Can you work these out from the model? Positions are in its coordinate system, mm. Face numbers are marked on the shaded views. A direction names the side the tool comes from. Round coordinates to 2 decimals unless told otherwise and drop trailing zeros. Loops run counter-clockwise (first coordinate to the right, second up) from the corner with the lowest first, then second, coordinate; pieces in that order, holes last. Notation, with made-up numbers: (-28.5, -22.75) -> (-23.5, -22.75) arc R9 cw to (-23.5, -5.75) -> close; hole circle Ø3 at (-34.75, 26.5). An arc over 180 degrees is marked (long way). Answer as a JSON object with one key per item and string values.
```python
from build123d import *

# Parameters (mm, degrees)
SKETCH2_W                = 12.7
SKETCH2_H                = 14.91
SKETCH2_R                = 5.08
BOSS_EXTRUDE1_DEPTH      = 9.525
BOSS_EXTRUDE2_START      = 9.525
BOSS_EXTRUDE2_DEPTH      = 6.35
BOSS_EXTRUDE3_DEPTH      = 2
BOSS_EXTRUDE7_START      = -25.4
BOSS_EXTRUDE7_DEPTH      = 50.8
SKETCH5_W                = 9.77111141
SKETCH5_H                = 3
CUT_EXTRUDE1_DEPTH       = 68.279429146
CUT_EXTRUDE2_START       = -12.902497
SKETCH6_W                = 30.31497918
SKETCH6_H                = 2.000002
SKETCH6_W_2              = 22.73097918
SKETCH6_H_2              = 6.646875
CUT_EXTRUDE2_DEPTH       = 12.902497
CUT_EXTRUDE3_START       = 0.499999
SKETCH6_3_W              = 22.73097918
SKETCH6_3_H              = 2.000002
SKETCH6_3_H_2            = 4.646873
SKETCH6_3_W_2            = 0.271399
SKETCH6_3_H_3            = 3
CUT_EXTRUDE3_DEPTH       = 7.0000114
FILLET2_R                = 17.78
CUT_EXTRUDE4_DEPTH       = 33.871006443
CUT_EXTRUDE4_DEPTH_BACK  = 33.871006443
SKETCH7_W                = 10.16
SKETCH7_H                = 10.092503778
FILLET3_R                = 2.54
SKETCH8_W                = 1.515
SKETCH8_H                = 2.54
BOSS_EXTRUDE8_DEPTH      = 2
FILLET4_R                = 5.08
CUT_EXTRUDE5_DEPTH       = 35.535859512
BOSS_EXTRUDE9_DEPTH      = 3.646875
SET_SCREW_CUT_REACH      = 43.018
SET_SCREW_CUT_END_RADIUS = 5.08
SKETCH12_R               = 1.4


# Read off the part's stored shape, not the designer's step: Boss-Extrude7
with BuildPart() as part:
    # Sketch2 → Boss-Extrude1 (new body)
    with BuildSketch(Plane.XY):
        with Locations((0, 7.455)):
            Rectangle(SKETCH2_W, SKETCH2_H)
        with Locations(Location((0, 7.83, 0), (0, 0, 180))):
            Circle(SKETCH2_R, mode=Mode.SUBTRACT)
    extrude(amount=BOSS_EXTRUDE1_DEPTH)

    # Sketch2<3> → Boss-Extrude2 (add)
    with BuildSketch(Plane.XY.offset(BOSS_EXTRUDE2_START)):
        Polygon((2.286, 0), (-2.286, 0), (-2.286, -5.334), (-4.826, -5.334), (-4.826, -14.859), (4.826, -14.859), (4.826, -5.334), (2.286, -5.334), align=None)
    extrude(amount=-BOSS_EXTRUDE2_DEPTH)

    # Sketch3 → Boss-Extrude3 (add)
    with BuildSketch(Plane.XZ):
        Polygon((14.9225, 9.525), (-14.9225, 9.525), (-14.9225, -11.557), (-10.85748959, -11.557), (10.85748959, -11.557), (14.9225, -11.557), align=None)
    extrude(amount=-BOSS_EXTRUDE3_DEPTH)

    # Boss-Extrude7 outline → Boss-Extrude7 (add)
    with BuildSketch(Plane(origin=(0, 0, 0), x_dir=(0, 0, -1), z_dir=(1, 0, 0)).offset(BOSS_EXTRUDE7_START)):
        with BuildLine():
            Line((5.848505491, 2), (11.557, 0))
            Line((11.557, 0), (12.724273166, 0.598024588))
            ThreePointArc((12.724273166, 0.598024588), (12.796184179, 0.55223881), (12.869936616, 0.509482413))
            Line((12.869936616, 0.509482413), (20.955, 3.646875))
            Line((20.955, 3.646875), (23.495, 3.646875))
            Line((23.495, 3.646875), (23.495, 6.646875))
            Line((23.495, 6.646875), (17.823506348, 6.646875))
            Line((17.823506348, 6.646875), (5.848505491, 2))
        make_face()
    extrude(amount=BOSS_EXTRUDE7_DEPTH)

    # Sketch5 → Cut-Extrude1 (cut, through all)
    with BuildSketch(Plane(origin=(0, 37.971305566, -23.495), x_dir=(1, 0, 0), z_dir=(0, 0, 1))):
        Polygon((25.4, -37.971305566), (25.4, -34.324430566), (15.62888859, -34.324430566), (14.9225, -34.324430566), (14.9225, -37.971305566), align=None)
        with Locations((20.514444295, -32.824430566)):
            Rectangle(SKETCH5_W, SKETCH5_H)
        Polygon((-25.4, -34.324430566), (-25.4, -37.971305566), (-14.9225, -37.971305566), (-14.9225, -34.324430566), (-15.62888859, -34.324430566), align=None)
        with Locations((-20.514444295, -32.824430566)):
            Rectangle(SKETCH5_W, SKETCH5_H)
    extrude(amount=CUT_EXTRUDE1_DEPTH, mode=Mode.SUBTRACT)

    # Sketch6 → Cut-Extrude2 (cut)
    with BuildSketch(Plane(origin=(0, 0, -22.995001), x_dir=(-1, 0, 0), z_dir=(0, 0, -1)).offset(CUT_EXTRUDE2_START)):
        with Locations((0, 5.646874)):
            Rectangle(SKETCH6_W, SKETCH6_H)
        with Locations((0, 3.3234375)):
            Rectangle(SKETCH6_W_2, SKETCH6_H_2)
    extrude(amount=CUT_EXTRUDE2_DEPTH, mode=Mode.SUBTRACT)

    # Sketch6<3> → Cut-Extrude3 (cut)
    with BuildSketch(Plane(origin=(0, 0, -22.995001), x_dir=(-1, 0, 0), z_dir=(0, 0, -1)).offset(CUT_EXTRUDE3_START)):
        with Locations((0, 5.646874)):
            Rectangle(SKETCH6_3_W, SKETCH6_3_H)
        with Locations((0, 2.3234365)):
            Rectangle(SKETCH6_3_W, SKETCH6_3_H_2)
        with Locations((-15.49318909, 5.146875)):
            Rectangle(SKETCH6_3_W_2, SKETCH6_3_H_3)
        with Locations((15.49318909, 5.146875)):
            Rectangle(SKETCH6_3_W_2, SKETCH6_3_H_3)
    extrude(amount=-CUT_EXTRUDE3_DEPTH, mode=Mode.SUBTRACT)

    # Fillet2
    fillet2_edges = [part.edges().sort_by_distance(p)[0] for p in [
        (0, 2, -5.848505491),
    ]]
    fillet(fillet2_edges, radius=FILLET2_R)

    # Sketch7 → Cut-Extrude4 (cut, two sides: drawn at the far end of the back side and taken through both)
    with BuildSketch(Plane(origin=(0, 2, 0), x_dir=(1, 0, 0), z_dir=(0, 1, 0)).offset(-CUT_EXTRUDE4_DEPTH_BACK)):
        with Locations((0, 5.046251889)):
            Rectangle(SKETCH7_W, SKETCH7_H)
    extrude(amount=CUT_EXTRUDE4_DEPTH + CUT_EXTRUDE4_DEPTH_BACK, mode=Mode.SUBTRACT)

    # Fillet3
    # the kernel refuses this fillet: 2.54 mm, written as the material it adds along each edge
    with BuildSketch(Plane(origin=(-5.08, 2, 0), x_dir=(1, 0, 0), z_dir=(0, -1, 0))) as fillet3_piece_1:
        with BuildLine():
            CenterArc((FILLET3_R, -FILLET3_R), FILLET3_R, 90, 90)
            Line((0, -FILLET3_R), (-FILLET3_R * 0.02, -FILLET3_R))
            Line((-FILLET3_R * 0.02, -FILLET3_R), (-FILLET3_R * 0.02, FILLET3_R * 0.02))
            Line((-FILLET3_R * 0.02, FILLET3_R * 0.02), (FILLET3_R, FILLET3_R * 0.02))
            Line((FILLET3_R, FILLET3_R * 0.02), (FILLET3_R, 0))
        make_face()
    extrude(amount=2)
    with BuildSketch(Plane(origin=(5.08, 0, 0), x_dir=(0, 0, -1), z_dir=(0, 1, 0))) as fillet3_piece_2:
        with BuildLine():
            CenterArc((FILLET3_R, FILLET3_R), FILLET3_R, 180, 90)
            Line((0, FILLET3_R), (-FILLET3_R * 0.02, FILLET3_R))
            Line((-FILLET3_R * 0.02, FILLET3_R), (-FILLET3_R * 0.02, -FILLET3_R * 0.02))
            Line((-FILLET3_R * 0.02, -FILLET3_R * 0.02), (FILLET3_R, -FILLET3_R * 0.02))
            Line((FILLET3_R, -FILLET3_R * 0.02), (FILLET3_R, 0))
        make_face()
    extrude(amount=2)

    # Sketch8 → Boss-Extrude8 (add)
    with BuildSketch(Plane(origin=(0, 4.646873, 0), x_dir=(1, 0, 0), z_dir=(0, 1, 0))):
        with Locations((-14.39998959, 17.915001)):
            Rectangle(SKETCH8_W, SKETCH8_H)
        with Locations((14.39998959, 17.915001)):
            Rectangle(SKETCH8_W, SKETCH8_H)
    extrude(amount=BOSS_EXTRUDE8_DEPTH)

    # Fillet4
    fillet4_edges = [part.edges().sort_by_distance(p)[0] for p in [
        (11.36548959, 1.823437543, -10.092504),
        (-11.36548959, 1.823437543, -10.092504),
    ]]
    fillet(fillet4_edges, radius=FILLET4_R)

    # Sketch10 → Cut-Extrude5 (cut, through all)
    with BuildSketch(Plane(origin=(4.826, 0, 0), x_dir=(0, 0, -1), z_dir=(1, 0, 0))):
        with BuildLine():
            Line((-6.243675471, -13.842705282), (-9.525, -5.334))
            Line((-9.525, -5.334), (-9.525, -14.859))
            Line((-9.525, -14.859), (-4.7625, -14.859))
            ThreePointArc((-4.7625, -14.859), (-5.660655851, -14.580496684), (-6.243675471, -13.842705282))
        make_face()
        with BuildLine():
            ThreePointArc((-3.175, -13.2715), (-3.639967985, -14.394032015), (-4.7625, -14.859))
            Line((-4.7625, -14.859), (-3.175, -14.859))
            Line((-3.175, -14.859), (-3.175, -13.2715))
        make_face()
    extrude(amount=-CUT_EXTRUDE5_DEPTH, mode=Mode.SUBTRACT)

    # Sketch11 → Boss-Extrude9 (add)
    with BuildSketch(Plane.XZ.offset(-3.646875)):
        with BuildLine():
            Line((11.36548959, -20.955), (11.36548959, -15.172503778))
            ThreePointArc((11.36548959, -15.172503778), (11.225613574, -13.98862244), (10.8136884, -12.869936616))
            Line((10.8136884, -12.869936616), (10.8136884, -10.092503778))
            Line((10.8136884, -10.092503778), (14.9225, -10.092503778))
            Line((14.9225, -10.092503778), (15.62888859, -10.092503778))
            Line((15.62888859, -10.092503778), (15.62888859, -16.4949886))
            Line((15.62888859, -16.4949886), (15.35748959, -16.4949886))
            Line((15.35748959, -16.4949886), (15.35748959, -23.495))
            Line((15.35748959, -23.495), (11.36548959, -23.495))
            Line((11.36548959, -23.495), (11.36548959, -20.955))
        make_face()
        with BuildLine():
            Line((-14.9225, -10.092503778), (-10.8136884, -10.092503778))
            Line((-10.8136884, -10.092503778), (-10.8136884, -12.869936616))
            ThreePointArc((-10.8136884, -12.869936616), (-11.225613574, -13.98862244), (-11.36548959, -15.172503778))
            Line((-11.36548959, -15.172503778), (-11.36548959, -20.955))
            Line((-11.36548959, -20.955), (-11.36548959, -23.495))
            Line((-11.36548959, -23.495), (-15.35748959, -23.495))
            Line((-15.35748959, -23.495), (-15.35748959, -16.4949886))
            Line((-15.35748959, -16.4949886), (-15.62888859, -16.4949886))
            Line((-15.62888859, -16.4949886), (-15.62888859, -10.092503778))
            Line((-15.62888859, -10.092503778), (-14.9225, -10.092503778))
        make_face()
    extrude(amount=BOSS_EXTRUDE9_DEPTH)

    # Set Screw Cut: up to this cylinder (the profile starts outside it)
    set_screw_cut_end = Plane(origin=(0, 7.83, 4.7625), z_dir=(0, 0, -1)) * Cylinder(SET_SCREW_CUT_END_RADIUS, 97.196, mode=Mode.PRIVATE)
    # Sketch12 → Set Screw Cut (cut, up to the surface)
    with BuildSketch(Plane(origin=(0, 14.91, 0), x_dir=(1, 0, 0), z_dir=(0, 1, 0)), mode=Mode.PRIVATE) as set_screw_cut_sk1:
        with Locations(Location((0, -4.7625, 0), (0, 0, 180))):
            Circle(SKETCH12_R)
    set_screw_cut_tool1 = extrude(set_screw_cut_sk1.sketch, amount=-SET_SCREW_CUT_REACH, mode=Mode.PRIVATE) - set_screw_cut_end
    add(set_screw_cut_tool1.solids().sort_by_distance((0, 14.91, 4.7625))[0], mode=Mode.SUBTRACT)


solid = part.part
```
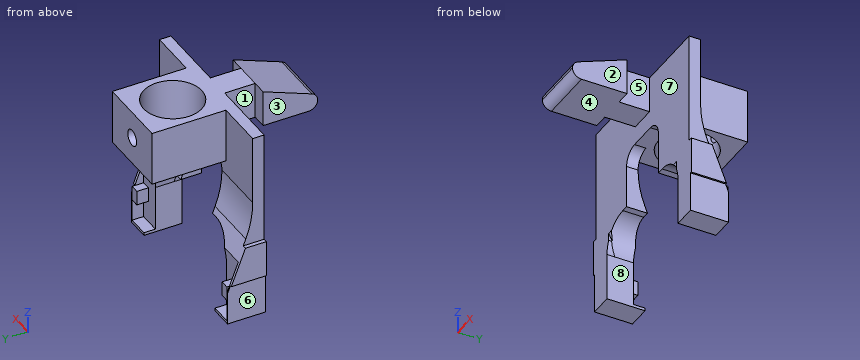
Q1. We'd pull the mould along X, two halves only. Please class the marked faces 6, 7 and 8: pulls with the +X half, pulls with the -X half, needs draft (parallel to the pull), parting line crosses it, or undercut.
Determined:
{"face 6": "pulls with the -X half", "face 7": "needs draft", "face 8": "undercut"}
Q2. I'm going to push flat-ended pins straight in: pin 1 (2 mm diameter, centred on x = 12.5, z = -19.5, fed in from +Y); pin 2 (10 mm diameter, centred on x = -6, y = 6.5, fed in from -Z); pin 3 (4 mm diameter, centred on y = -9, z = 6, fed in from -X); pin 4 (5 mm diameter, centred on y = -4.5, z = -13.5, fed in from -X). Where does each tip first touch, or does it pass through?
Determined:
{"pin 1": "y = 4.65", "pin 2": "z = -12.53", "pin 3": "x = -4.83", "pin 4": "through"}
Q3. I want a section at B-B, the plane x = 0. Give the number of separate pieces and of enclosed holes in the cut face, then the cut area to 3 significant figures.
Determined:
{"separate pieces": "3", "enclosed holes": "0", "area": "116 mm²"}
Q4. I want a section at A-A, the plane y = 7.83. Write out the boundary of the cut face in (x, z) (3 decimals), then the cut area to 3 significant figures.
Determined:
{"outline": "(-6.35, 0) -> (-5.08, 0) -> (-5.08, 9.525) -> (-6.35, 9.525) -> close; (5.08, 0) -> (6.35, 0) -> (6.35, 9.525) -> (5.08, 9.525) -> close", "area": "24.2 mm²"}
Q5. On a 3-axis mill with a long thin cutter (end or side, diameter ignored), from which of +Z, -Z, +X, -X, +Y, -Y can I reach the whole of each face in a straight line? I mean the marked faces 1, 2, 3, 4 and 5. Say none if no direction works.
Determined:
{"face 1": "+Z, -Z, -X", "face 2": "+Z, -Z, +X, -Y", "face 3": "+Z, -Z, -X, -Y", "face 4": "-Z, +X, -X, -Y", "face 5": "+Z, -Z, +X"}
Q6. I want a section at C-C, the plane z = -1.5. Write out the boundary of the cut face in (x, y), then the cut area to 3 significant figures.
Determined:
{"outline": "(-14.92, 0) -> (-4.86, 0) -> (-4.86, 2) -> (-14.92, 2) -> close; (4.86, 0) -> (14.92, 0) -> (14.92, 2) -> (4.86, 2) -> close", "area": "40.3 mm²"}
Q7. If I drill on L1, parallel to Z at x = 0, y = 13.6 (1 decimal); L2, parallel to X at y = 2, z = -17; L3, parallel to Y at x = 11, z = 6.5, over which ranges is the centre line in solid material (lowest first)? Write a range as [from, to].
Determined:
{"L1": "[0, 3.4], [6.2, 9.5]", "L2": "[-15.36, -11.37], [11.37, 15.36]", "L3": "[0, 2]"}
Q8. I want a section at D-D, the plane x = 13. Write out the boundary of the cut face in (y, z) (1 decimal).
Determined:
{"outline": "(0, -23.5) -> (6.6, -23.5) -> (6.6, -23) -> (4.6, -23) -> (4.6, -12.7) -> (3.2, -9) arc R17.8 cw to (2, -2.5) -> (2, 9.5) -> (0, 9.5) -> close"}
